```python
from build123d import *

# Parameters (mm, degrees)
SKETCH1_R           = 2.4892
SKETCH1_R_2         = 2.4511
SKETCH1_R_3         = 7.62
SKETCH1_R_4         = 14.2875
BOSS_EXTRUDE1_DEPTH = 2.54
FILLET1_R           = 7.62


with BuildPart() as part:
    # Sketch1 → Boss-Extrude1 (new body)
    with BuildSketch(Plane.XY):
        with BuildLine():
            Line((-76.2, -15.1892), (-76.2, -25.4))
            Line((-76.2, -25.4), (76.2, -25.4))
            Line((76.2, -25.4), (76.2, -15.1892))
            ThreePointArc((76.2, -15.1892), (73.7108, -12.7), (76.2, -10.2108))
            Line((76.2, -10.2108), (76.2, 133.35))
            Line((76.2, 133.35), (-76.2, 133.35))
            Line((-76.2, 133.35), (-76.2, -10.2108))
            ThreePointArc((-76.2, -10.2108), (-73.7108, -12.7), (-76.2, -15.1892))
        make_face()
        with Locations((-63.5, -12.7)):
            Circle(SKETCH1_R, mode=Mode.SUBTRACT)
        with Locations((-50.8, -12.7)):
            Circle(SKETCH1_R, mode=Mode.SUBTRACT)
        with Locations((-38.1, -12.7)):
            Circle(SKETCH1_R, mode=Mode.SUBTRACT)
        with Locations((-50.8, 6.705273841)):
            Circle(SKETCH1_R_2, mode=Mode.SUBTRACT)
        with Locations((-25.4, -12.7)):
            Circle(SKETCH1_R, mode=Mode.SUBTRACT)
        with Locations((-12.7, -12.7)):
            Circle(SKETCH1_R, mode=Mode.SUBTRACT)
        with Locations((-25.4, 6.705273841)):
            Circle(SKETCH1_R_2, mode=Mode.SUBTRACT)
        with Locations((-63.5, 28.702319097)):
            Circle(SKETCH1_R_2, mode=Mode.SUBTRACT)
        with Locations((-38.1, 28.702319097)):
            Circle(SKETCH1_R_3, mode=Mode.SUBTRACT)
        with Locations((-50.8, 50.699364354)):
            Circle(SKETCH1_R_2, mode=Mode.SUBTRACT)
        with Locations((-12.7, 28.702319097)):
            Circle(SKETCH1_R_2, mode=Mode.SUBTRACT)
        with Locations((-25.4, 50.699364354)):
            Circle(SKETCH1_R_2, mode=Mode.SUBTRACT)
        with Locations((0, -12.7)):
            Circle(SKETCH1_R, mode=Mode.SUBTRACT)
        with Locations((12.7, -12.7)):
            Circle(SKETCH1_R, mode=Mode.SUBTRACT)
        with Locations((25.4, -12.7)):
            Circle(SKETCH1_R, mode=Mode.SUBTRACT)
        with Locations((25.4, 6.705273841)):
            Circle(SKETCH1_R_2, mode=Mode.SUBTRACT)
        with Locations((38.1, -12.7)):
            Circle(SKETCH1_R, mode=Mode.SUBTRACT)
        with Locations((50.8, -12.7)):
            Circle(SKETCH1_R, mode=Mode.SUBTRACT)
        with Locations((63.5, -12.7)):
            Circle(SKETCH1_R, mode=Mode.SUBTRACT)
        with Locations((50.8, 6.705273841)):
            Circle(SKETCH1_R_2, mode=Mode.SUBTRACT)
        with Locations((12.7, 28.702319097)):
            Circle(SKETCH1_R_2, mode=Mode.SUBTRACT)
        with Locations((0, 53.975)):
            Circle(SKETCH1_R_4, mode=Mode.SUBTRACT)
        with Locations((25.4, 50.699364354)):
            Circle(SKETCH1_R_2, mode=Mode.SUBTRACT)
        with Locations((38.1, 28.702319097)):
            Circle(SKETCH1_R_3, mode=Mode.SUBTRACT)
        with Locations((63.5, 28.702319097)):
            Circle(SKETCH1_R_2, mode=Mode.SUBTRACT)
        with Locations((50.8, 50.699364354)):
            Circle(SKETCH1_R_2, mode=Mode.SUBTRACT)
        with Locations((0, 109.855)):
            Circle(SKETCH1_R_4, mode=Mode.SUBTRACT)
    extrude(amount=BOSS_EXTRUDE1_DEPTH)

    # Fillet1
    fillet1_edges = [part.edges().sort_by_distance(p)[0] for p in [
        (-76.2, 133.35, 1.27),
        (76.2, 133.35, 1.27),
        (76.2, -25.4, 1.27),
        (-76.2, -25.4, 1.27),
    ]]
    fillet(fillet1_edges, radius=FILLET1_R)


solid = part.part
```
The listing builds one solid part. Answer for the finished solid, in the listing's coordinates (mm). Round coordinates to 2 decimals unless told otherwise and drop trailing zeros. Order: outer loops, then holes, each group sorted by start corner. A loop starts at its lowest first (then second) coordinate and runs counter-clockwise, first axis right, second up. Notation, with made-up numbers: (57, 50) - (98, 50) arc R33 cw to (98, 84) - close; hole circle Ø5 at (-15.5, -18.5). An arc over 180 degrees is marked (long way). Put each result on its own line as item: value. Start each with the question number.
(1) Straight lines are drawn through the part: probe 1 along X at (y, z) = (7, 2); probe 2 along Y at (x, z) = (25.4, 1.65); probe 3 along Y at (x, z) = (63.5, 0.9). For each, find the intervals that lie inside material, in ascending order. Write a range as from..to.
(2) Find section A-A (x = 0). Give the vertices of the cut face in (y, z), plus the area to 3 significant figures.
(3) Find section C-C (x = -63.5). Give the vertices of the cut face in (y, z), plus the area to 3 significant figures.
(4) Determine the mould class of faces 1 (the cylindrical face through (73.909, -23.227, 1.288)), 2 (the cylindrical face through (12.17, 26.31, 1.25)), 3 (the flat face through (16, 55, 0)) for opening direction X: released by +X, released by -X, zero draft, split by the parting line, or undercut.
(5) Find section D-D (y = 101). Give the vertices of the cut face in (x, z).
(6) Find section B-B (y = 119). Give the vertices of the cut face in (x, z), plus the area to 3 significant figures.
Reply:
1. probe 1: -76.2..-53.23, -48.37..-27.83, -22.97..22.97, 27.83..48.37, 53.23..76.2
1. probe 2: -25.4..-15.19, -10.21..4.25, 9.16..48.25, 53.15..133.35
1. probe 3: -25.4..-15.19, -10.21..26.25, 31.15..133.35
2. outline: (-25.4, 0) - (-15.19, 0) - (-15.19, 2.54) - (-25.4, 2.54) - close; (-10.21, 0) - (39.69, 0) - (39.69, 2.54) - (-10.21, 2.54) - close; (68.26, 0) - (95.57, 0) - (95.57, 2.54) - (68.26, 2.54) - close; (124.14, 0) - (133.35, 0) - (133.35, 2.54) - (124.14, 2.54) - close
2. area: 245 mm^2
3. outline: (-25.4, 0) - (-15.19, 0) - (-15.19, 2.54) - (-25.4, 2.54) - close; (-10.21, 0) - (26.25, 0) - (26.25, 2.54) - (-10.21, 2.54) - close; (31.15, 0) - (133.35, 0) - (133.35, 2.54) - (31.15, 2.54) - close
3. area: 378 mm^2
4. face 1: released by +X
4. face 2: undercut
4. face 3: zero draft
5. outline: (-76.2, 0) - (-11.21, 0) - (-11.21, 2.54) - (-76.2, 2.54) - close; (11.21, 0) - (76.2, 0) - (76.2, 2.54) - (11.21, 2.54) - close
6. outline: (-76.2, 0) - (-10.98, 0) - (-10.98, 2.54) - (-76.2, 2.54) - close; (10.98, 0) - (76.2, 0) - (76.2, 2.54) - (10.98, 2.54) - close
6. area: 331 mm^2
